Could you check a few things on this drawing? It's one solid part, dimensions in mm from its lowest x, y, z. Give positions to 0.01 mm unless a question says otherwise; leave off trailing zeros. Loops run counter-clockwise (first coordinate to the right, second up) from the corner with the lowest first, then second, coordinate; pieces in that order, holes last. Notation, with made-up numbers: M -33.75,32.25 L 17.25,32.25 A18 cw 17.25,50.25 Z; hole C -25.75,-15 d9. An arc over 180 degrees is marked long. Answer as CSV lines item,"result". Start each with the question number.
Item 1: If I drill on line 1 along X through (y, z) = (3.25, 10); line 2 along X through (y, z) = (3.75, 9); line 3 along Z through (x, y) = (45, 4.25), over which ranges is the centre line in solid material (lowest first)? Write a range as from..to.
Item 2: I want a section at D-D on x = 7. List the corners of the cut face in (y, z) for me.
Item 3: If we mould it in two halves opening along X, with no side actions, what happens to the marked faces 1, 2 and 3? For each: released by +X, released by -X, zero draft, split by the parting line, or undercut.
Item 4: I want a section at A-A on z = 10. List the corners of the cut face in (x, y) for me.
Item 5: I want a section at C-C on y = 1.5. List the corners of the cut face in (x, z) for me, plus the area to 3 significant figures.
Item 6: I want a section at B-B on x = 23. List the corners of the cut face in (y, z) for me, plus the area to 3 significant figures.
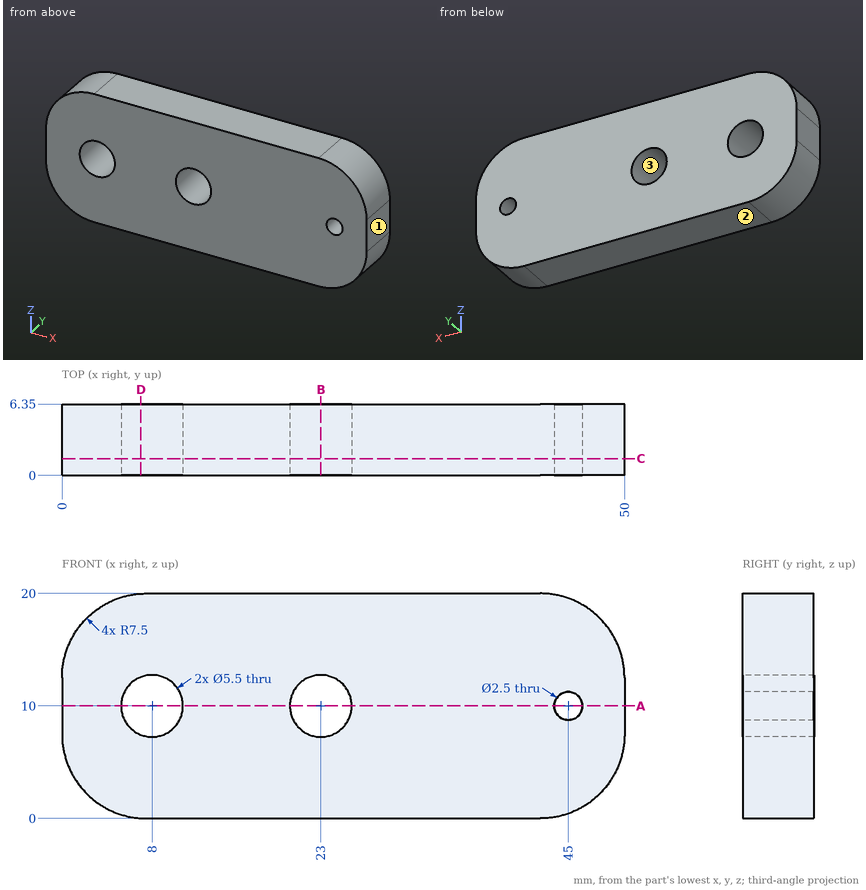
Result:
1,line 1,"0..5.25, 10.75..20.25, 25.75..43.75, 46.25..50"
1,line 2,"0..5.44, 10.56..20.44, 25.56..44.25, 45.75..50"
1,line 3,"0.43..8.75, 11.25..19.57"
2,outline,"M 0,0.02 L 6.35,0.02 L 6.35,7.44 L 0,7.44 Z; M 0,12.56 L 6.35,12.56 L 6.35,19.98 L 0,19.98 Z"
3,face 1,"released by +X"
3,face 2,"zero draft"
3,face 3,"undercut"
4,outline,"M 0,0 L 5.25,0 L 5.25,6.35 L 0,6.35 Z; M 10.75,0 L 20.25,0 L 20.25,6.35 L 10.75,6.35 Z; M 25.75,0 L 43.75,0 L 43.75,6.35 L 25.75,6.35 Z; M 46.25,0 L 50,0 L 50,6.35 L 46.25,6.35 Z"
5,outline,"M 0,7.5 A7.5 ccw 7.5,0 L 42.5,0 A7.5 ccw 50,7.5 L 50,12.5 A7.5 ccw 42.5,20 L 7.5,20 A7.5 ccw 0,12.5 Z; hole C 8,10 d5.5; hole C 23,10 d5.5; hole C 45,10 d2.5"
5,area,"899 mm^2"
6,outline,"M 0,0 L 6.35,0 L 6.35,7.25 L 0,7.25 Z; M 0,12.75 L 6.35,12.75 L 6.35,20 L 0,20 Z"
6,area,"92.1 mm^2"
